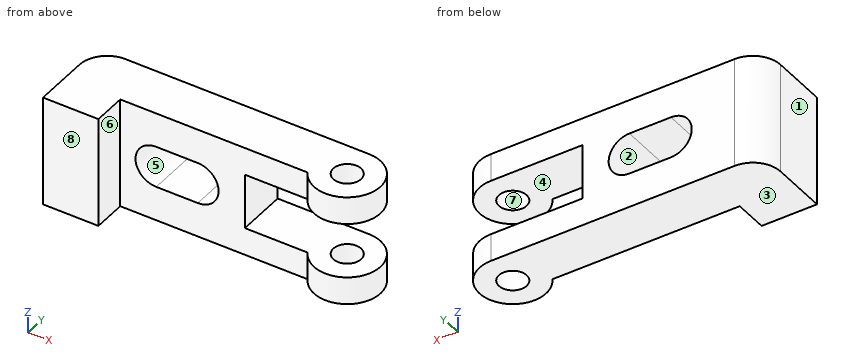
```python
from build123d import *

# Parameters (mm, degrees)
ESQUISSE1_R             = 50
BOSS_EXTRU_1_DEPTH      = 400
ESQUISSE2_W             = 600
ESQUISSE2_H             = 200
ENL_V_MAT_EXTRU_1_DEPTH = 1209.304597359


with BuildPart() as part:
    # Esquisse1 → Boss.-Extru.1 (new body)
    with BuildSketch(Plane.XY):
        with BuildLine():
            Line((0, 0), (0, 200))
            ThreePointArc((0, 200), (29.289321881, 270.710678119), (100, 300))
            Line((100, 300), (980, 300))
            ThreePointArc((980, 300), (1083.923048454, 120), (876.076951546, 120))
            Line((876.076951546, 120), (200, 120))
            Line((200, 120), (200, 0))
            Line((200, 0), (0, 0))
        make_face()
        with Locations((980, 180)):
            Circle(ESQUISSE1_R, mode=Mode.SUBTRACT)
    extrude(amount=BOSS_EXTRU_1_DEPTH)

    # Esquisse2 → Enlèv. mat.-Extru.1 (cut, through all)
    with BuildSketch(Plane(origin=(0, 300, 0), x_dir=(1, 0, 0), z_dir=(0, 1, 0))):
        with BuildLine():
            Line((330, -125), (480, -125))
            ThreePointArc((480, -125), (555, -200), (480, -275))
            Line((480, -275), (330, -275))
            ThreePointArc((330, -275), (255, -200), (330, -125))
        make_face()
        with Locations((950, -200)):
            Rectangle(ESQUISSE2_W, ESQUISSE2_H)
    extrude(amount=-ENL_V_MAT_EXTRU_1_DEPTH, mode=Mode.SUBTRACT)


solid = part.part
```
Geometry: final body of the model. Coordinates: model frame, mm. Face numbers are marked on the shaded views. A direction names the side the tool comes from. Round coordinates to 2 decimals unless told otherwise and drop trailing zeros. Order: outer loops, then holes, each group sorted by start corner. A loop starts at its lowest first (then second) coordinate and runs counter-clockwise, first axis right, second up. Notation, with made-up numbers: (61, 24.25) -> (100, 24.25) arc R26 ccw to (100, 47.25) -> close; hole circle Ø7 at (14.25, -10). An arc over 180 degrees is marked (long way). Use one line per item in the form item = value.
(1) Section B-B on z = 338.5. Return loops of the section in (x, y), and give its area (3 significant figures).
Results list:
outline = (0, 0) -> (200, 0) -> (200, 120) -> (876.08, 120) arc R120 ccw (long way) to (980, 300) -> (100, 300) arc R100 ccw to (0, 200) -> close; hole circle Ø100 at (980, 180)
area = 217,000 mm^2
(2) Access query for the marked faces 4, 5, 6, 7 and 8. Directions: +Z, -Z, +X, -X, +Y, -Y. A direction counts if a zero-diameter tool reaches every point of the face in a straight line with its end or side. Return the directions, or none.
Results list:
face_4 = +X, +Y, -Y
face_5 = +Y, -Y
face_6 = +Z, -Z, -Y
face_7 = +Z, -Z
face_8 = +Z, -Z, +X, -X, -Y
(3) Ray query, probe 1 along Z at (x, y) = (671.5, 194); probe 2 along Z at (x, y) = (430, 183); probe 3 along X at (y, z) = (180, 353). Return the intervals inside material, ascending. Write a range as [from, to].
Results list:
probe_1 = [0, 100], [300, 400]
probe_2 = [0, 125], [275, 400]
probe_3 = [0, 930], [1030, 1100]
(4) Draft query along Z for the marked faces 1, 2 and 3. Return one class per face: pulls with the +Z half, pulls with the -Z half, needs draft (parallel to the pull), parting line crosses it, or undercut.
Results list:
face_1 = needs draft
face_2 = undercut
face_3 = pulls with the -Z half
(5) Section D-D on z = 166.5. Return loops of the section in (x, y).
Results list:
outline = (0, 0) -> (200, 0) -> (200, 120) -> (262.9, 120) -> (262.9, 300) -> (100, 300) arc R100 ccw to (0, 200) -> close; (547.1, 120) -> (650, 120) -> (650, 300) -> (547.1, 300) -> close
(6) Section A-A on y = 180. Return loops of the section in (x, z), and give its area (3 significant figures).
Results list:
outline = (0, 0) -> (930, 0) -> (930, 100) -> (650, 100) -> (650, 300) -> (930, 300) -> (930, 400) -> (0, 400) -> close; (1030, 0) -> (1100, 0) -> (1100, 100) -> (1030, 100) -> close; (1030, 300) -> (1100, 300) -> (1100, 400) -> (1030, 400) -> close; hole (330, 125) -> (480, 125) arc R75 ccw to (480, 275) -> (330, 275) arc R75 ccw to start
area = 290,000 mm^2
(7) First-contact query: pin 1 Ø1 at (y, z) = (112, 315) entering from +X. Flat tip, straight axial feed; report the tip coordinate or a pass-through.
Results list:
pin_1 = 1079.22
(8) Section C-C on x = 439.5. Return loops of the section in (y, z).
Results list:
outline = (120, 0) -> (300, 0) -> (300, 125) -> (120, 125) -> close; (120, 275) -> (300, 275) -> (300, 400) -> (120, 400) -> close
